Could you check a few things on this model? Use its own coordinates, in mm. A direction names the side the tool comes from. Round coordinates to 2 decimals unless told otherwise and drop trailing zeros. Write each loop counter-clockwise with the first axis right and the second up, starting at its lowest first coordinate (ties: lowest second). Pieces come first, ordered by that corner, then holes. Notation, with made-up numbers: (32.25, 6) -> (37.25, 6) arc R19 ccw to (37.25, 41) -> close; hole circle Ø1 at (48, 56). An arc over 180 degrees is marked (long way). Answer in a Markdown table with one row per item.
from build123d import *

# Parameters (mm, degrees)
BOSS_EXTRUDE1_DEPTH = 45
SKETCH3_R           = 8.255
CUT_EXTRUDE1_DEPTH  = 7.35
SKETCH2_3_W         = 38.649999916
SKETCH2_3_H         = 38.649999916
BOSS_EXTRUDE2_DEPTH = 5.08
SKETCH4_R           = 8.255
CUT_EXTRUDE2_DEPTH  = 7.35
FILLET1_R           = 2.54


with BuildPart() as part:
    # Sketch2 → Boss-Extrude1 (new body)
    with BuildSketch(Plane(origin=(0, 0, 0), x_dir=(0, 0, -1), z_dir=(1, 0, 0))):
        Polygon((44.999999916, 6.35), (6.35, 6.35), (6.35, 44.999999916), (0, 44.999999916), (0, 0), (44.999999916, 0), align=None)
    extrude(amount=BOSS_EXTRUDE1_DEPTH)

    # Sketch3 → Cut-Extrude1 (cut, through all)
    with BuildSketch(Plane(origin=(0, 6.35, 0), x_dir=(1, 0, 0), z_dir=(0, 1, 0))):
        with Locations((22.5, 22.499999958)):
            Circle(SKETCH3_R)
    extrude(amount=-CUT_EXTRUDE1_DEPTH, mode=Mode.SUBTRACT)

    # Sketch2_3 → Boss-Extrude2 (add)
    with BuildSketch(Plane(origin=(0, 0, 0), x_dir=(0, 0, -1), z_dir=(1, 0, 0))):
        with Locations((25.674999958, 25.674999958)):
            Rectangle(SKETCH2_3_W, SKETCH2_3_H)
    extrude(amount=BOSS_EXTRUDE2_DEPTH)

    # Sketch4 → Cut-Extrude2 (cut, through all)
    with BuildSketch(Plane(origin=(0, 0, -6.35), x_dir=(-1, 0, 0), z_dir=(0, 0, -1))):
        with Locations((-22.5, 22.499999958)):
            Circle(SKETCH4_R)
    extrude(amount=-CUT_EXTRUDE2_DEPTH, mode=Mode.SUBTRACT)

    # Fillet1
    fillet1_edges = [part.edges().sort_by_distance(p)[0] for p in [
        (22.5, 0, 0),
        (25.04, 6.35, -6.35),
        (45, 44.999999916, -3.175),
        (2.54, 44.999999916, -44.999999916),
        (5.08, 25.674999958, -6.35),
        (5.08, 6.35, -25.674999958),
        (45, 3.175, -44.999999916),
        (0, 0, -22.499999958),
        (0, 22.499999958, 0),
    ]]
    fillet(fillet1_edges, radius=FILLET1_R)


solid = part.part
1) Imagine slicing it at D-D, the plane z = -33. Please give me the cut outline in (x, y).
Findings:
| item | result |
|---|---|
| outline | (0, 2.54) arc R2.54 ccw to (2.54, 0) -> (45, 0) -> (45, 6.35) -> (7.62, 6.35) arc R2.54 cw to (5.08, 8.89) -> (5.08, 45) -> (0, 45) -> close |
2) Imagine slicing it at A-A, the plane z = -22.5. Please give me the cut outline in (x, y) (3 decimals).
Findings:
| item | result |
|---|---|
| outline | (0, 2.54) arc R2.54 ccw to (2.54, 0) -> (14.245, 0) -> (14.245, 6.35) -> (7.62, 6.35) arc R2.54 cw to (5.08, 8.89) -> (5.08, 45) -> (0, 45) -> close; (30.755, 0) -> (45, 0) -> (45, 6.35) -> (30.755, 6.35) -> close |
3) Thinking about a two-plate mould opening in Y: for faces 1 (the face through (24.067, 0.724, -0.764)), 2 (the face through (23.575, 30.685, -3.219)), 3 (the face through (0.724, 23.473, -0.764)), 4 (the face through (44.236, 44.276, -3.131)), which applies, +Y half, -Y half, draft (parallel to the pull), parting line (faces both ways), or undercut?
Findings:
| item | result |
|---|---|
| face 1 | -Y half |
| face 2 | undercut |
| face 3 | draft |
| face 4 | +Y half |
4) For pin 1 (10 mm diameter, centred on x = 22.5, z = -22.5, fed in from -Y); pin 2 (3 mm diameter, centred on x = 17.5, z = -39.5, fed in from +Y); pin 3 (8 mm diameter, centred on x = 24.5, z = -18.5, fed in from -Y); pin 4 (11 mm diameter, centred on x = 30, y = 30.5, fed in from -Z), each with a flat end and sliding along its axis, tell me the tip position at first contact or that it passes through.
Findings:
| item | result |
|---|---|
| pin 1 | passes through |
| pin 2 | stops at y = 6.35 |
| pin 3 | stops at y = 0 |
| pin 4 | stops at z = -6.35 |
5) Imagine slicing it at B-B, the plane y = 22.5. Please give me the cut outline in (x, z) (3 decimals).
Findings:
| item | result |
|---|---|
| outline | (0, -45) -> (5.08, -45) -> (5.08, -8.89) arc R2.54 cw to (7.62, -6.35) -> (14.245, -6.35) -> (14.245, 0) -> (2.54, 0) arc R2.54 ccw to (0, -2.54) -> close; (30.755, -6.35) -> (45, -6.35) -> (45, 0) -> (30.755, 0) -> close |
6) For faces 5 (the face through (26.572, 7.074, -7.114)), 6 (the face through (23, 0, -14)), which set-ups out of +Z, -Z, +X, -X, +Y, -Y let a thin tool reach every point of the face, with its end or its side?
Findings:
| item | result |
|---|---|
| face 5 | -Z, +X, +Y |
| face 6 | +Z, -Z, +X, -X, -Y |
7) Imagine slicing it at C-C, the plane x = 22.5. Please give me the cut outline in (y, z) (3 decimals).
Findings:
| item | result |
|---|---|
| outline | (0, -45) -> (6.35, -45) -> (6.35, -30.755) -> (0, -30.755) -> close; (0, -14.245) -> (6.35, -14.245) -> (6.35, -8.89) arc R2.54 cw to (8.89, -6.35) -> (14.245, -6.35) -> (14.245, 0) -> (2.54, 0) arc R2.54 ccw to (0, -2.54) -> close; (30.755, -6.35) -> (45, -6.35) -> (45, 0) -> (30.755, 0) -> close |
8) Please list where these lines run through material, in increasing order: line 1 (Y direction, x = 22, z = -3); line 2 (Z direction, x = 22.5, y = 3) (3 decimals); line 3 (Y direction, x = 22.5, z = -2.5) (3 decimals).
Findings:
| item | result |
|---|---|
| line 1 | y = 0 to 14.26, 30.74 to 45 |
| line 2 | z = -45 to -30.755, -14.245 to 0 |
| line 3 | y = 0 to 14.245, 30.755 to 45 |
